```python
from build123d import *

# Parameters (mm, degrees)
F1_DEPTH  = 12
F2_W      = 100
F2_H      = 20
F3_DEPTH  = 5
F4_W      = 135
F4_H      = 20
F5_DEPTH  = 5
F7_R      = 2.5
F8_DEPTH  = 25
F9_DEPTH  = 5
F10_W     = 20
F10_H     = 20
F10_W_2   = 100
F10_H_2   = 130
F11_DEPTH = 25
F12_W     = 130
F12_H     = 16
F13_DEPTH = 100.0010001


with BuildPart() as f1:
    # F0 (on Top) → F1 (new body)
    with BuildSketch(Plane.XY):
        with BuildLine():
            add(Edge.make_bspline(
                [(-86.5, 0), (-86.5, -116.5), (0, -116.5)],
                knots=[1.5707963268, 1.5707963268, 1.5707963268, 3.1415926536, 3.1415926536, 3.1415926536], degree=2, weights=[1, 0.7071067812, 1]))
            Line((-86.5, 0), (-86.5, -116.5))
            Line((-86.5, -116.5), (0, -116.5))
        make_face()
        Polygon((-86.5, -116.5), (-86.5, 0), (-100, 0), (-100, -130), (0, -130), (0, -116.5), align=None)
    extrude(amount=F1_DEPTH)

    # F2 (on face) → F3 (join)
    with BuildSketch(Plane.XZ.offset(130)):
        with Locations((-50, 6)):
            Rectangle(F2_W, F2_H)
    extrude(amount=F3_DEPTH)

    # F4 (on face) → F5 (join)
    with BuildSketch(Plane(origin=(-100, 0, 0), x_dir=(0, -1, 0), z_dir=(-1, 0, 0))):
        with Locations((67.5, 6)):
            Rectangle(F4_W, F4_H)
    extrude(amount=F5_DEPTH)

    # F7 (on face) → F8 (join)
    with BuildSketch(Plane(origin=(0, 0, -4), x_dir=(1, 0, 0), z_dir=(0, 0, -1))):
        Polygon((0, 135), (0, 150), (-120, 150), (-120, 0), (-105, 0), (-105, 135), align=None)
        with Locations((-110, 30)):
            Circle(F7_R, mode=Mode.SUBTRACT)
        with Locations((-110, 105)):
            Circle(F7_R, mode=Mode.SUBTRACT)
        with Locations((-80, 140)):
            Circle(F7_R, mode=Mode.SUBTRACT)
        with Locations((-30, 140)):
            Circle(F7_R, mode=Mode.SUBTRACT)
    extrude(amount=-F8_DEPTH)

    # F6 (on face) → F9 (join)
    with BuildSketch(Plane.XY.offset(16)):
        Polygon((-90, 0), (-105, 0), (-105, -135), (0, -135), (0, -120), (-90, -120), align=None)
    extrude(amount=F9_DEPTH)

    # F10 (on Top) → F11 (cut, symmetric)
    with BuildSketch(Plane.XY):
        with Locations((-10, -10)):
            Rectangle(F10_W, F10_H)
        with Locations((-70, -10)):
            Rectangle(F10_W_2, F10_H)
        with Locations((-10, -85)):
            Rectangle(F10_W, F10_H_2)
    extrude(amount=F11_DEPTH, both=True, mode=Mode.SUBTRACT)

    # F12 (on face) → F13 (cut, through all)
    with BuildSketch(Plane.YZ.offset(-20)):
        with Locations((-85, 4)):
            Rectangle(F12_W, F12_H)
    extrude(amount=-F13_DEPTH, mode=Mode.SUBTRACT)


solid = f1.part
```
CAD build for the part. Positions are in the model's coordinates, mm. A direction names the side the tool comes from. Round coordinates to 2 decimals unless told otherwise and drop trailing zeros. Write each loop counter-clockwise with the first axis right and the second up, starting at its lowest first coordinate (ties: lowest second). Pieces come first, ordered by that corner, then holes. Notation, with made-up numbers: (14.25, 17) - (64.25, 17) arc R10 ccw to (64.25, 28) - close; hole circle Ø5 at (81, -29.75). An arc over 180 degrees is marked (long way). Return JSON: item names as keys, results as strings. Group by question number.
Item 1: Band-saw the part on B-B on y = -30. List the corners of the cut face in (x, z), plus the area to 3 significant figures.
Item 2: 3-axis set-ups, long thin cutter, end or side, ignore diameter. For faces 1 (the face through (-90, -71, 18)), 2 (the face through (-20, -139, 17)), 3 (the face through (-100, -74, 14)): which of +Z, -Z, +X, -X, +Y, -Y reach the whole face in a straight line?
Item 3: Probe probe 1 along Y at (x, z) = (-110, 18.75); probe 2 along Y at (x, z) = (-80, 14.5); probe 3 along Y at (x, z) = (-108, 14.75). List the from-to ranges inside material, lowest first.
Item 4: Band-saw the part on C-C on z = 17.5. List the corners of the cut face in (x, y).
Item 5: Band-saw the part on D-D on y = -140. List the corners of the cut face in (x, z), plus the area to 3 significant figures.
Item 6: Mould opens along Y. For faces 4 (the face through (-30.33, -142.48, 16.44)), 5 (the face through (-69, -150, 16)), 6 (the face through (-107.615, -105.751, 16.437)), 7 (the face through (-109, -20, 17)) say: +Y half, -Y half, draft (parallel to the pull), parting line (faces both ways), or undercut.
Item 7: Flat gauge pins, fed straight in: pin 1 Ø4 at (y, z) = (-64, 19) entering from +X; pin 2 Ø1.5 at (x, y) = (-48, -125) entering from -Z; pin 3 Ø4 at (x, z) = (-33, 15) entering from +Y; pin 4 Ø6.5 at (x, y) = (-80, -140) entering from -Z. Where does each tip first touch, or does it go through?
Item 8: Band-saw the part on A-A on x = -80. List the corners of the cut face in (y, z).
Resolved:
{
 "1": {"outline": "(-120, 12) - (-112.5, 12) - (-112.5, 21) - (-120, 21) - close; (-107.5, 12) - (-100, 12) - (-100, 16) - (-90, 16) - (-90, 21) - (-107.5, 21) - close", "area": "185 mm²"},
 "2": {"face 1": "+Z, -Z, +X, +Y", "face 2": "+Z, -Z, +X, +Y, -Y", "face 3": "-Z, +X, +Y"},
 "3": {"probe 1": "y = -150 to -107.5, -102.5 to -32.5, -27.5 to -20", "probe 2": "y = -150 to -142.5, -137.5 to -130", "probe 3": "y = -150 to -106.5, -103.5 to -31.5, -28.5 to -20"},
 "4": {"outline": "(-120, -150) - (-20, -150) - (-20, -120) - (-90, -120) - (-90, -20) - (-120, -20) - close; hole circle Ø5 at (-110, -105); hole circle Ø5 at (-110, -30); hole circle Ø5 at (-80, -140); hole circle Ø5 at (-30, -140)"},
 "5": {"outline": "(-120, 12) - (-82.5, 12) - (-82.5, 21) - (-120, 21) - close; (-77.5, 12) - (-32.5, 12) - (-32.5, 21) - (-77.5, 21) - close; (-27.5, 12) - (-20, 12) - (-20, 21) - (-27.5, 21) - close", "area": "810 mm²"},
 "6": {"face 4": "undercut", "face 5": "-Y half", "face 6": "undercut", "face 7": "+Y half"},
 "7": {"pin 1": "stops at x = -90", "pin 2": "stops at z = 16", "pin 3": "stops at y = -120", "pin 4": "stops at z = 12"},
 "8": {"outline": "(-150, 12) - (-142.5, 12) - (-142.5, 21) - (-150, 21) - close; (-137.5, 12) - (-130, 12) - (-130, 16) - (-120, 16) - (-120, 21) - (-137.5, 21) - close"}
}
